Can you work these out from the model? Positions are in its coordinate system, mm. A direction names the side the tool comes from. Coordinates: 2 decimals unless noted, no trailing zeros. Order: outer loops, then holes, each group sorted by start corner. A loop starts at its lowest first (then second) coordinate and runs counter-clockwise, first axis right, second up. Notation, with made-up numbers: (-29.5, 1) -> (-21.5, 1) arc R29 cw to (-21.5, 38) -> close; hole circle Ø1 at (17.25, 60). An arc over 180 degrees is marked (long way). Answer as a JSON object with one key per item and string values. Group by question number.
(1) For pin 1 (1.1 mm diameter, centred on x = -48.5, z = 0.5, fed in from -Y); pin 2 (0.6 mm diameter, centred on x = -49, y = 6.5, fed in from +Z); pin 3 (0.8 mm diameter, centred on x = -48.5, z = 0.5, fed in from +Y), each with a flat end and sliding along its axis, tell me the tip position at first contact or that it passes through.
(2) Which directions (+Z, -Z, +X, -X, +Y, -Y) give clear straight access to the entire face, cutting with the end or side of a thin tool? Please do faces 4 (the flat face through (-49, -7, 1)), 5 (the flat face through (16, 8, 1)), 6 (the flat face through (10.175, -11, 1)).
(3) I want a section at C-C, the plane x = 13. List the corners of the cut face in (y, z) for me, plus the area to 3 significant figures.
(4) I want a section at A-A, the plane z = 1.4. List the corners of the cut face in (x, y) for me.
(5) I need wall thicknesses on line 1 (Y direction, x = 15, z = 1.15); line 2 (X direction, y = -9, z = 1.05); line 3 (X direction, y = -1, z = 0.5). Which ranges of each line are inside material? Lowest first, please.
(6) I want a section at B-B, the plane y = 0.5. List the corners of the cut face in (x, z) for me.
(7) If we mould it in two halves opening along Y, with no side actions, what happens to faces 1 (the flat face through (10.175, 11, 1)), 2 (the cylindrical face through (23.574, -7.43, 1.014)), 3 (the flat face through (-18, 15.75, 1))? For each: pulls with the +Y half, pulls with the -Y half, needs draft (parallel to the pull), parting line crosses it, or undercut.
from build123d import *

# Parameters (mm, degrees)
F0_W     = 14
F0_H     = 16
F1_DEPTH = 2
F0_W_2   = 2
F0_H_2   = 8
F2_DEPTH = 1
F3_R     = 2


with BuildPart() as f1:
    # F0 (on Top) → F1 (new body)
    with BuildSketch(Plane.XY):
        Polygon((-47.824564, -15.75), (10.175436, -15.75), (10.175436, -8), (-3.824564, -8), (-3.824564, 8), (10.175436, 8), (10.175436, 15.75), (-47.824564, 15.75), (-47.824564, 10.75), (-47.824564, 2.75), (-47.824564, -2.75), (-47.824564, -10.75), align=None)
        with Locations((3.175436, 0)):
            Rectangle(F0_W, F0_H)
        with Locations((17.175436, 0)):
            Rectangle(F0_W, F0_H)
    extrude(amount=F1_DEPTH)

    # F0 (on Top) → F2 (join)
    with BuildSketch(Plane.XY):
        with Locations((-48.824564, 6.75)):
            Rectangle(F0_W_2, F0_H_2)
        with Locations((-48.824564, -6.75)):
            Rectangle(F0_W_2, F0_H_2)
    extrude(amount=F2_DEPTH)

    # F3
    f3_edges = [f1.edges().sort_by_distance(p)[0] for p in [
        (10.175436, 15.75, 1),
        (24.175436, 8, 1),
        (24.175436, -8, 1),
        (10.175436, -15.75, 1),
        (-47.824564, -15.75, 1),
        (-47.824564, 15.75, 1),
    ]]
    fillet(f3_edges, radius=F3_R)


solid = f1.part
Computed values:
{
 "1": {"pin 1": "stops at y = -10.75", "pin 2": "stops at z = 1", "pin 3": "stops at y = 10.75"},
 "2": {"face 4": "+Z, -X, +Y, -Y", "face 5": "+Z, -Z, +X, +Y", "face 6": "+Z, -Z, +X, -Y"},
 "3": {"outline": "(-8, 0) -> (8, 0) -> (8, 2) -> (-8, 2) -> close", "area": "32.0 mm2"},
 "4": {"outline": "(-47.82, -13.75) arc R2 ccw to (-45.82, -15.75) -> (8.18, -15.75) arc R2 ccw to (10.18, -13.75) -> (10.18, -8) -> (22.18, -8) arc R2 ccw to (24.18, -6) -> (24.18, 6) arc R2 ccw to (22.18, 8) -> (10.18, 8) -> (10.18, 13.75) arc R2 ccw to (8.18, 15.75) -> (-45.82, 15.75) arc R2 ccw to (-47.82, 13.75) -> close"},
 "5": {"line 1": "y = -8 to 8", "line 2": "x = -47.82 to 10.18", "line 3": "x = -47.82 to 24.18"},
 "6": {"outline": "(-47.82, 0) -> (24.18, 0) -> (24.18, 2) -> (-47.82, 2) -> close"},
 "7": {"face 1": "needs draft", "face 2": "pulls with the -Y half", "face 3": "pulls with the +Y half"}
}
